```python
from build123d import *

# Parameters (mm, degrees)
F0_R     = 11
F1_DEPTH = 7


with BuildPart() as f1:
    # F0 (on Top) → F1 (new body)
    with BuildSketch(Plane.XY):
        Polygon((0, 50), (-10.606602, 25.606602), (-35.355339, 35.355339), (-25.606602, 10.606602), (-50, 0), (-25.606602, -10.606602), (-35.355339, -35.355339), (-10.606602, -25.606602), (0, -50), (10.606602, -25.606602), (35.355339, -35.355339), (25.606602, -10.606602), (50, 0), (25.606602, 10.606602), (35.355339, 35.355339), (10.606602, 25.606602), align=None)
        Polygon((7.252651, -24.896849), (0, -41.576724), (-7.252651, -24.896849), (-3.311682, -24.896849), (-3.311682, -15.702289), (0, -15.702289), (3.311682, -15.702289), (3.311682, -24.896849), align=None, mode=Mode.SUBTRACT)
        Polygon((-12.476332, -22.733129), (-29.399184, -29.399184), (-22.733129, -12.476332), (-19.946444, -15.263018), (-13.444908, -8.761482), (-11.103195, -11.103195), (-8.761482, -13.444908), (-15.263018, -19.946444), align=None, mode=Mode.SUBTRACT)
        Polygon((22.733129, -12.476332), (29.399184, -29.399184), (12.476332, -22.733129), (15.263018, -19.946444), (8.761482, -13.444908), (11.103195, -11.103195), (13.444908, -8.761482), (19.946444, -15.263018), align=None, mode=Mode.SUBTRACT)
        Polygon((-24.896849, -7.252651), (-41.576724, 0), (-24.896849, 7.252651), (-24.896849, 3.311682), (-15.702289, 3.311682), (-15.702289, 0), (-15.702289, -3.311682), (-24.896849, -3.311682), align=None, mode=Mode.SUBTRACT)
        Polygon((-22.733129, 12.476332), (-29.399184, 29.399184), (-12.476332, 22.733129), (-15.263018, 19.946444), (-8.761482, 13.444908), (-11.103195, 11.103195), (-13.444908, 8.761482), (-19.946444, 15.263018), align=None, mode=Mode.SUBTRACT)
        Circle(F0_R, mode=Mode.SUBTRACT)
        Polygon((12.476332, 22.733129), (29.399184, 29.399184), (22.733129, 12.476332), (19.946444, 15.263018), (13.444908, 8.761482), (11.103195, 11.103195), (8.761482, 13.444908), (15.263018, 19.946444), align=None, mode=Mode.SUBTRACT)
        Polygon((24.896849, 7.252651), (41.576724, 0), (24.896849, -7.252651), (24.896849, -3.311682), (15.702289, -3.311682), (15.702289, 0), (15.702289, 3.311682), (24.896849, 3.311682), align=None, mode=Mode.SUBTRACT)
        Polygon((-7.252651, 24.896849), (0, 41.576724), (7.252651, 24.896849), (3.311682, 24.896849), (3.311682, 15.702289), (0, 15.702289), (-3.311682, 15.702289), (-3.311682, 24.896849), align=None, mode=Mode.SUBTRACT)
    extrude(amount=F1_DEPTH)


solid = f1.part
```
CAD build for the part. Positions are in the model's coordinates, mm. A direction names the side the tool comes from. Round coordinates to 2 decimals unless told otherwise and drop trailing zeros. Write each loop counter-clockwise with the first axis right and the second up, starting at its lowest first coordinate (ties: lowest second). Pieces come first, ordered by that corner, then holes. Notation, with made-up numbers: (52.5, 77) - (100.5, 77) arc R10 cw to (100.5, 95) - close; hole circle Ø7 at (68, 79.25). An arc over 180 degrees is marked (long way). Return JSON: item names as keys, results as strings. Group by question number.
Item 1: Band-saw the part on A-A on x = 36.5. List the corners of the cut face in (y, z), plus the area to 3 significant figures.
Item 2: Band-saw the part on C-C on z = 2.5. State how many separate pieces and enclosed holes the cut face has, plus the area to 3 significant figures.
Item 3: Band-saw the part on B-B on y = 17.5. List the corners of the cut face in (x, z).
Item 4: Band-saw the part on D-D on y = 38.5. List the corners of the cut face in (x, z).
Item 5: Probe probe 1 along X at (y, z) = (16.5, 3.75); probe 2 along Y at (x, z) = (-13, 4.25); probe 3 along X at (y, z) = (-13.5, 3). List the from-to ranges inside material, lowest first.
Item 6: 3-axis set-ups, long thin cutter, end or side, ignore diameter. For faces 5 (the face through (5.38, 37.63, 3.45)), 6 (the face through (37.97, 5.23, 3.45)), 7 (the face through (-37.97, -5.23, 3.45)), 8 (the face through (-3.677, 33.12, 3.451)), 9 (the face through (-4, -11, 0)): which of +Z, -Z, +X, -X, +Y, -Y reach the whole face in a straight line?
Item 7: Flat gauge pins, fed straight in: pin 1 Ø2 at (x, z) = (-20, 4.5) entering from +Y; pin 2 Ø3 at (y, z) = (5, 3) entering from -X; pin 3 Ø1.2 at (y, z) = (-5.5, 4.5) entering from +X; pin 4 Ø8 at (x, y) = (2, 20) entering from -Z. Where does each tip first touch, or does it go through?
Item 8: Mould opens along Y. For faces 1 (the face through (30.549, -23.154, 3.451)), 2 (the face through (20.82, 26.02, 3.45)), 3 (the face through (-22.808, 30.413, 3.451)), 4 (the face through (22.808, -30.413, 3.451)) say: +Y half, -Y half, draft (parallel to the pull), parting line (faces both ways), or undercut.
Resolved:
{
 "1": {"outline": "(-5.87, 0) - (-2.21, 0) - (-2.21, 7) - (-5.87, 7) - close; (2.21, 0) - (5.87, 0) - (5.87, 7) - (2.21, 7) - close", "area": "51.3 mm²"},
 "2": {"separate pieces": "1", "enclosed holes": "9", "area": "2,410 mm²"},
 "3": {"outline": "(-28.32, 0) - (-24.71, 0) - (-24.71, 7) - (-28.32, 7) - close; (-12.82, 0) - (-3.31, 0) - (-3.31, 7) - (-12.82, 7) - close; (3.31, 0) - (12.82, 0) - (12.82, 7) - (3.31, 7) - close; (24.71, 0) - (28.32, 0) - (28.32, 7) - (24.71, 7) - close"},
 "4": {"outline": "(-5, 0) - (-1.34, 0) - (-1.34, 7) - (-5, 7) - close; (1.34, 0) - (5, 0) - (5, 7) - (1.34, 7) - close"},
 "5": {"probe 1": "x = -27.93 to -24.32, -11.82 to -3.31, 3.31 to 11.82, 24.32 to 27.93", "probe 2": "y = -26.55 to -22.94, -22.21 to -17.68, -9.21 to 9.21, 17.68 to 22.21, 22.94 to 26.55", "probe 3": "x = -26.75 to -23.14, -21.71 to -18.18, -8.82 to 8.82, 18.18 to 21.71, 23.14 to 26.75"},
 "6": {"face 5": "+Z, -Z, +Y", "face 6": "+Z, -Z, +X", "face 7": "+Z, -Z, -X", "face 8": "+Z, -Z", "face 9": "-Z, +X, -X, +Y, -Y"},
 "7": {"pin 1": "stops at y = 29.7", "pin 2": "stops at x = -41.95", "pin 3": "stops at x = 38.73", "pin 4": "stops at z = 0"},
 "8": {"face 1": "undercut", "face 2": "undercut", "face 3": "+Y half", "face 4": "-Y half"}
}
